Build history of the part. All positions in model axes, mm. Face numbers are marked on the shaded views. A direction names the side the tool comes from. Give positions to 0.01 mm unless a question says otherwise; leave off trailing zeros. Order: outer loops, then holes, each group sorted by start corner. A loop starts at its lowest first (then second) coordinate and runs counter-clockwise, first axis right, second up. Notation, with made-up numbers: M 12,81 L 23,81 A26 cw 23,102 Z; hole C 27,79.25 d7. An arc over 180 degrees is marked long. Use CSV: the item, a comma, the result in double quotes. Start each with the question number.
Item 1: Band-saw the part on B-B on y = 11.5. Write the cut outline in (x, z), plus the area to 3 significant figures.
Item 2: Pin check, flat tips, straight feed: P1, Ø6, axis at x = 6.5, y = 12, coming from the +Z side; P2, Ø2, axis at x = 4.5, y = 7.5, coming from the -Z side; P3, Ø1, axis at x = 29.5, y = 12, coming from the -Z side. Stop position of each tip, or through.
Item 3: Which spindle directions (+Z, -Z, +X, -X, +Y, -Y) get a long thin tool onto all of the face, cutting with end or side? Do the marked faces 4 and 5. Say none if no direction does.
Item 4: Band-saw the part on C-C on z = 10. Write the cut outline in (x, y).
Item 5: Band-saw the part on A-A on z = 1.35. Write the cut outline in (x, y).
Item 6: Two-plate mould, pull along X, no slides. Class the marked faces 1, 2 and 3: pulls with the +X half, pulls with the -X half, needs draft (parallel to the pull), parting line crosses it, or undercut.
Item 7: Band-saw the part on D-D on x = 10. Write the cut outline in (y, z).
Item 8: Wall check: line 1 along X through (y, z) = (0.8, 18.65); line 2 along Z through (x, y) = (43.6, 0.55); line 3 along Y through (x, z) = (26, 18). Give the ranges that are in metal, low to high.
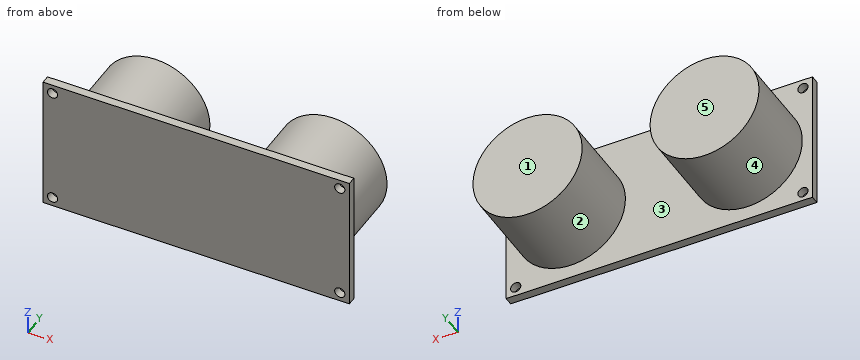
from build123d import *

# Parameters (mm, degrees)
SKETCH1_W           = 45
SKETCH1_H           = 20
SKETCH1_R           = 0.75
BOSS_EXTRUDE1_DEPTH = 1.25
SKETCH3_R           = 8
BOSS_EXTRUDE2_DEPTH = 12
SKETCH4_R           = 8.018104591
BOSS_EXTRUDE3_DEPTH = 12


with BuildPart() as part:
    # Sketch1 → Boss-Extrude1 (new body)
    with BuildSketch(Plane(origin=(0, 0, 0), x_dir=(1, 0, 0), z_dir=(0, 1, 0))):
        with Locations((22.5, -10)):
            Rectangle(SKETCH1_W, SKETCH1_H)
        with Locations(Location((1.4, -18.65, 0), (0, 0, 270))):
            Circle(SKETCH1_R, mode=Mode.SUBTRACT)
        with Locations(Location((1.4, -1.35, 0), (0, 0, 90))):
            Circle(SKETCH1_R, mode=Mode.SUBTRACT)
        with Locations(Location((43.6, -18.65, 0), (0, 0, 90))):
            Circle(SKETCH1_R, mode=Mode.SUBTRACT)
        with Locations(Location((43.6, -1.35, 0), (0, 0, 270))):
            Circle(SKETCH1_R, mode=Mode.SUBTRACT)
    extrude(amount=BOSS_EXTRUDE1_DEPTH)

    # Sketch3 → Boss-Extrude2 (add)
    with BuildSketch(Plane(origin=(0, 1.25, 0), x_dir=(1, 0, 0), z_dir=(0, 1, 0))):
        with Locations(Location((9.5, -10, 0), (0, 0, 270))):
            Circle(SKETCH3_R)
    extrude(amount=BOSS_EXTRUDE2_DEPTH)

    # Sketch4 → Boss-Extrude3 (add)
    with BuildSketch(Plane(origin=(0, 1.25, 0), x_dir=(1, 0, 0), z_dir=(0, 1, 0))):
        with Locations(Location((35.5, -10, 0), (0, 0, 270))):
            Circle(SKETCH4_R)
    extrude(amount=BOSS_EXTRUDE3_DEPTH)


solid = part.part
Model answer:
1,outline,"C 9.5,10 d16; C 35.5,10 d16.04"
1,area,"403 mm^2"
2,P1,"stops at z = 18"
2,P2,"stops at z = 3.07"
2,P3,"stops at z = 4.17"
3,face 4,"+Y"
3,face 5,"+Z, -Z, +X, -X, +Y"
4,outline,"M 0,0 L 45,0 L 45,1.25 L 43.52,1.25 L 43.52,13.25 L 27.48,13.25 L 27.48,1.25 L 17.5,1.25 L 17.5,13.25 L 1.5,13.25 L 1.5,1.25 L 0,1.25 Z"
5,outline,"M 0,0 L 0.65,0 L 0.65,1.25 L 0,1.25 Z; M 2.15,0 L 42.85,0 L 42.85,1.25 L 2.15,1.25 Z; M 44.35,0 L 45,0 L 45,1.25 L 44.35,1.25 Z"
6,face 1,"needs draft"
6,face 2,"undercut"
6,face 3,"undercut"
7,outline,"M 0,0 L 1.25,0 L 1.25,2.02 L 13.25,2.02 L 13.25,17.98 L 1.25,17.98 L 1.25,20 L 0,20 Z"
8,line 1,"x = 0 to 0.65, 2.15 to 42.85, 44.35 to 45"
8,line 2,"z = 0 to 0.6, 2.1 to 17.9, 19.4 to 20"
8,line 3,"y = 0 to 1.25"
